Source: CAD feature listing. Evaluate the final solid. Frame: model axes, mm. Face numbers are marked on the shaded views. A direction names the side the tool comes from. Coordinates: 2 decimals unless noted, no trailing zeros. Write each loop counter-clockwise with the first axis right and the second up, starting at its lowest first coordinate (ties: lowest second). Pieces come first, ordered by that corner, then holes. Notation, with made-up numbers: (46.5, -8.75) -> (50.5, -8.75) arc R31 cw to (50.5, 18.25) -> close; hole circle Ø1 at (45, 52.25). An arc over 180 degrees is marked (long way). Write item = value, one per line.
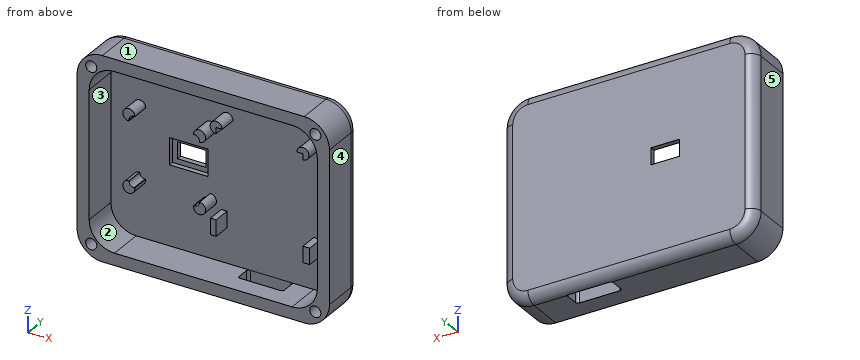
from build123d import *

# Parameters (mm, degrees)
BOSS_EXTRUDE1_DEPTH = 9
FILLET1_R           = 2
CUT_EXTRUDE1_DEPTH  = 7
SKETCH3_R           = 1.1
CUT_EXTRUDE2_DEPTH  = 6
SKETCH4_W           = 5.6
SKETCH4_H           = 3.3
CUT_EXTRUDE3_DEPTH  = 46.366235587
SKETCH5_W           = 7.6
SKETCH5_H           = 5.3
CUT_EXTRUDE4_DEPTH  = 1
SKETCH6_R           = 1.2
BOSS_EXTRUDE2_DEPTH = 3.5
CUT_EXTRUDE5_DEPTH  = 3.5
SKETCH9_R           = 1.2
SKETCH9_W           = 1.831616398
SKETCH9_H           = 3.192245721
SKETCH9_W_2         = 1.831616397
BOSS_EXTRUDE3_DEPTH = 3.5
SKETCH10_W          = 17.2
SKETCH10_H          = 21.10187295
CUT_EXTRUDE7_DEPTH  = 3.5
CUT_EXTRUDE8_DEPTH  = 3.5


with BuildPart() as part:
    # Sketch1 → Boss-Extrude1 (new body)
    with BuildSketch(Plane(origin=(0, 0, 0), x_dir=(1, 0, 0), z_dir=(0, 1, 0))):
        with BuildLine():
            Line((-34.540816327, 21.109693878), (5.459183673, 21.109693878))
            ThreePointArc((5.459183673, 21.109693878), (8.994717579, 19.645227783), (10.459183673, 16.109693878))
            Line((10.459183673, 16.109693878), (10.459183673, -13.890306122))
            ThreePointArc((10.459183673, -13.890306122), (8.994717579, -17.425840028), (5.459183673, -18.890306122))
            Line((5.459183673, -18.890306122), (-34.540816327, -18.890306122))
            ThreePointArc((-34.540816327, -18.890306122), (-38.076350232, -17.425840028), (-39.540816327, -13.890306122))
            Line((-39.540816327, -13.890306122), (-39.540816327, 16.109693878))
            ThreePointArc((-39.540816327, 16.109693878), (-38.076350232, 19.645227783), (-34.540816327, 21.109693878))
        make_face()
    extrude(amount=BOSS_EXTRUDE1_DEPTH)

    # Fillet1
    fillet1_edges = [part.edges().sort_by_distance(p)[0] for p in [
        (8.994717579, 9, -19.645227783),
        (-14.540816327, 9, -21.109693878),
        (-38.076350232, 9, -19.645227783),
        (-39.540816327, 9, -1.109693878),
        (-38.076350232, 9, 17.425840028),
        (-14.540816327, 9, 18.890306122),
        (8.994717579, 9, 17.425840028),
        (10.459183673, 9, -1.109693878),
    ]]
    fillet(fillet1_edges, radius=FILLET1_R)

    # Sketch2 → Cut-Extrude1 (cut)
    with BuildSketch(Plane.XZ):
        with BuildLine():
            Line((-32.140816327, 16.490306122), (3.059183673, 16.490306122))
            ThreePointArc((3.059183673, 16.490306122), (6.594717579, 15.025840028), (8.059183673, 11.490306122))
            Line((8.059183673, 11.490306122), (8.059183673, -13.709693878))
            ThreePointArc((8.059183673, -13.709693878), (6.594717579, -17.245227783), (3.059183673, -18.709693878))
            Line((3.059183673, -18.709693878), (-32.140816327, -18.709693878))
            ThreePointArc((-32.140816327, -18.709693878), (-35.676350232, -17.245227783), (-37.140816327, -13.709693878))
            Line((-37.140816327, -13.709693878), (-37.140816327, 11.490306122))
            ThreePointArc((-37.140816327, 11.490306122), (-35.676350232, 15.025840028), (-32.140816327, 16.490306122))
        make_face()
    extrude(amount=-CUT_EXTRUDE1_DEPTH, mode=Mode.SUBTRACT)

    # Sketch3 → Cut-Extrude2 (cut)
    with BuildSketch(Plane.XZ):
        with Locations(Location((7.659183673, 16.090306122, 0), (0, 0, 270))):
            Circle(SKETCH3_R)
        with Locations(Location((-36.740816327, 16.090306122, 0), (0, 0, 270))):
            Circle(SKETCH3_R)
        with Locations(Location((-36.740816327, -18.309693878, 0), (0, 0, 270))):
            Circle(SKETCH3_R)
        with Locations(Location((7.659183673, -18.309693878, 0), (0, 0, 270))):
            Circle(SKETCH3_R)
    extrude(amount=-CUT_EXTRUDE2_DEPTH, mode=Mode.SUBTRACT)

    # Sketch4 → Cut-Extrude3 (cut, through all)
    with BuildSketch(Plane.XZ.offset(-7)):
        with Locations((-21.740816327, -0.359693878)):
            Rectangle(SKETCH4_W, SKETCH4_H)
    extrude(amount=-CUT_EXTRUDE3_DEPTH, mode=Mode.SUBTRACT)

    # Sketch5 → Cut-Extrude4 (cut)
    with BuildSketch(Plane.XZ.offset(-7)):
        with Locations((-21.740816327, -0.359693878)):
            Rectangle(SKETCH5_W, SKETCH5_H)
    extrude(amount=-CUT_EXTRUDE4_DEPTH, mode=Mode.SUBTRACT)

    # Sketch6 → Boss-Extrude2 (add)
    with BuildSketch(Plane.XZ.offset(-7)):
        with Locations(Location((-17.440816327, 6.640306122, 0), (0, 0, 270))):
            Circle(SKETCH6_R)
        with Locations(Location((-31.440816327, 6.640306122, 0), (0, 0, 270))):
            Circle(SKETCH6_R)
        with Locations(Location((-31.440816327, -7.359693878, 0), (0, 0, 270))):
            Circle(SKETCH6_R)
        with Locations(Location((-17.440816327, -7.359693878, 0), (0, 0, 270))):
            Circle(SKETCH6_R)
    extrude(amount=BOSS_EXTRUDE2_DEPTH)

    # Sketch7 → Cut-Extrude5 (cut)
    with BuildSketch(Plane.XZ.offset(-3.5)):
        with BuildLine():
            Line((-30.440816327, 6.640306122), (-18.440816327, 6.640306122))
            ThreePointArc((-18.440816327, 6.640306122), (-17.733709545, 6.347412904), (-17.440816327, 5.640306122))
            Line((-17.440816327, 5.640306122), (-17.440816327, -6.206359886))
            ThreePointArc((-17.440816327, -6.206359886), (-17.733709545, -6.913466667), (-18.440816327, -7.206359886))
            Line((-18.440816327, -7.206359886), (-30.440816327, -7.206359886))
            ThreePointArc((-30.440816327, -7.206359886), (-31.147923108, -6.913466667), (-31.440816327, -6.206359886))
            Line((-31.440816327, -6.206359886), (-31.440816327, 5.640306122))
            ThreePointArc((-31.440816327, 5.640306122), (-31.147923108, 6.347412904), (-30.440816327, 6.640306122))
        make_face()
    extrude(amount=-CUT_EXTRUDE5_DEPTH, mode=Mode.SUBTRACT)

    # Sketch9 → Boss-Extrude3 (add)
    with BuildSketch(Plane.XZ.offset(-7)):
        with Locations(Location((3.059183673, 9.290306122, 0), (0, 0, 270))):
            Circle(SKETCH9_R)
        with Locations(Location((-14.140816327, 9.290306122, 0), (0, 0, 270))):
            Circle(SKETCH9_R)
        with Locations((-14.344094184, -10.215443968)):
            Rectangle(SKETCH9_W, SKETCH9_H)
        with Locations((3.487522214, -10.215443968)):
            Rectangle(SKETCH9_W_2, SKETCH9_H)
    extrude(amount=BOSS_EXTRUDE3_DEPTH)

    # Sketch10 → Cut-Extrude7 (cut)
    with BuildSketch(Plane.XZ.offset(-3.5)):
        with Locations((-5.540816327, -1.260630353)):
            Rectangle(SKETCH10_W, SKETCH10_H)
    extrude(amount=-CUT_EXTRUDE7_DEPTH, mode=Mode.SUBTRACT)

    # Sketch11 → Cut-Extrude8 (cut)
    with BuildSketch(Plane.XY.offset(-18.709693878)):
        with BuildLine():
            Line((-9.540816327, 7.15), (-1.540816327, 7.15))
            ThreePointArc((-1.540816327, 7.15), (-1.187262936, 7.003553391), (-1.040816327, 6.65))
            Line((-1.040816327, 6.65), (-1.040816327, 4.25))
            ThreePointArc((-1.040816327, 4.25), (-1.187262936, 3.896446609), (-1.540816327, 3.75))
            Line((-1.540816327, 3.75), (-9.540816327, 3.75))
            ThreePointArc((-9.540816327, 3.75), (-9.894369717, 3.896446609), (-10.040816327, 4.25))
            Line((-10.040816327, 4.25), (-10.040816327, 6.65))
            ThreePointArc((-10.040816327, 6.65), (-9.894369717, 7.003553391), (-9.540816327, 7.15))
        make_face()
    extrude(amount=-CUT_EXTRUDE8_DEPTH, mode=Mode.SUBTRACT)


solid = part.part
1) Reachability of the marked faces 1 and 2 from +Z, -Z, +X, -X, +Y, -Y: full face, straight path, thin tool, end or side. Return the list, or none.
Answer block:
face_1 = +Z, +X, -X, +Y, -Y
face_2 = -Y
2) Cut plane A-A, the plane x = -21.5. Output: boundary loops of the cut face in (y, z).
Answer block:
outline = (0, -21.11) -> (7, -21.11) arc R2 ccw to (9, -19.11) -> (9, -2.01) -> (8, -2.01) -> (8, -3.01) -> (7, -3.01) -> (7, -18.71) -> (0, -18.71) -> close; (0, 16.49) -> (7, 16.49) -> (7, 2.29) -> (8, 2.29) -> (8, 1.29) -> (9, 1.29) -> (9, 16.89) arc R2 ccw to (7, 18.89) -> (0, 18.89) -> close
3) Pull-direction query (X, two-part tool) for the marked faces 3, 4 and 5; classes: +X half, -X half, draft (parallel to the pull), parting line (faces both ways), or undercut.
Answer block:
face_3 = undercut
face_4 = +X half
face_5 = -X half
4) Cut plane D-D, the plane z = -9.5. Output: boundary loops of the cut face in (x, y), and give its area (3 significant figures).
Answer block:
outline = (-39.54, 0) -> (-37.14, 0) -> (-37.14, 7) -> (-15.26, 7) -> (-15.26, 3.5) -> (-14.14, 3.5) -> (-14.14, 7) -> (3.06, 7) -> (3.06, 3.5) -> (4.4, 3.5) -> (4.4, 7) -> (8.06, 7) -> (8.06, 0) -> (10.46, 0) -> (10.46, 7) arc R2 ccw to (8.46, 9) -> (-37.54, 9) arc R2 ccw to (-39.54, 7) -> close
area = 141 mm2
5) Cut plane B-B, the plane z = -1. Output: boundary loops of the cut face in (x, y).
Answer block:
outline = (-39.54, 0) -> (-37.14, 0) -> (-37.14, 7) -> (-25.54, 7) -> (-25.54, 8) -> (-24.54, 8) -> (-24.54, 9) -> (-37.54, 9) arc R2 ccw to (-39.54, 7) -> close; (-18.94, 8) -> (-17.94, 8) -> (-17.94, 7) -> (8.06, 7) -> (8.06, 0) -> (10.46, 0) -> (10.46, 7) arc R2 ccw to (8.46, 9) -> (-18.94, 9) -> close
6) First-contact query: pin 1 Ø12 at (x, z) = (-19.5, 2) entering from -Y; pin 2 Ø3 at (x, z) = (-5, 6.5) entering from -Y; pin 3 Ø0.7 at (y, z) = (5, -19.5) entering from -X. Flat tips, straight axial feed; report the tip coordinate or a pass-through.
Answer block:
pin_1 = 3.5
pin_2 = 7
pin_3 = -38.51
7) Cut plane C-C, the plane x = -29.5. Output: boundary loops of the cut face in (y, z).
Answer block:
outline = (0, -21.11) -> (7, -21.11) arc R2 ccw to (9, -19.11) -> (9, 16.89) arc R2 ccw to (7, 18.89) -> (0, 18.89) -> (0, 16.49) -> (7, 16.49) -> (7, -18.71) -> (0, -18.71) -> close
8) Material intervals for probe 1 along X at (y, z) = (5.25, -11.5); probe 2 along Z at (x, y) = (-1, 4.75); probe 3 along X at (y, z) = (4.5, 0), sorted ascending. Write a range as [from, to].
Answer block:
probe_1 = [-39.54, -37.14], [-15.26, -14.14], [3.06, 4.4], [8.06, 10.46]
probe_2 = [-21.11, -18.71], [16.49, 18.89]
probe_3 = [-39.54, -37.14], [8.06, 10.46]
